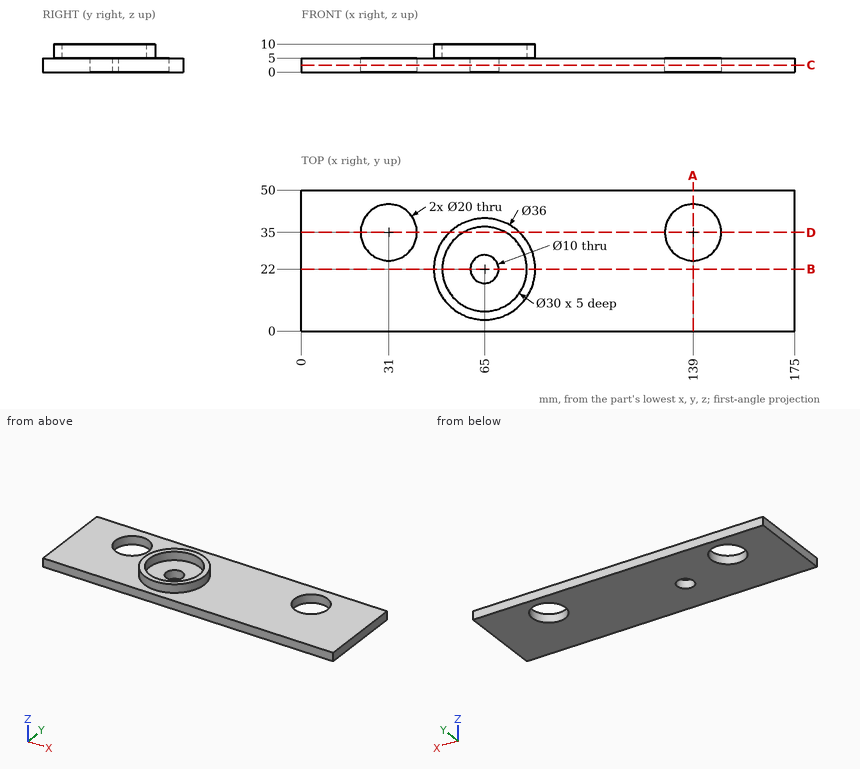
Check sheet for the drawn part. Datum: minimum x, y, z corner. Units: mm. Coordinates: 2 decimals unless noted, no trailing zeros. Write each loop counter-clockwise with the first axis right and the second up, starting at its lowest first coordinate (ties: lowest second). Pieces come first, ordered by that corner, then holes. Notation, with made-up numbers: M 49,-13.75 L 93,-13.75 A12 cw 93,4.25 Z; hole C 40.5,-6.5 d2. An arc over 180 degrees is marked long. One line per item, written item: value.
Item 1: Scan lines: line 1 along Y through (x, z) = (139, 3.75); line 2 along X through (y, z) = (21, 9.75); line 3 along Z through (x, y) = (72, 44.5). Record each from-to range of solid material in increasing order.
Check sheet entries:
line 1: y = 0 to 25, 45 to 50
line 2: x = 47.03 to 50.03, 79.97 to 82.97
line 3: z = 0 to 5
Item 2: Section check C-C, the plane z = 2.5. Record the boundary of the cut face in (x, y).
Check sheet entries:
outline: M 0,0 L 175,0 L 175,50 L 0,50 Z; hole C 31,35 d20; hole C 65,22 d10; hole C 139,35 d20
Item 3: Section check B-B, the plane y = 22. Record the boundary of the cut face in (x, z).
Check sheet entries:
outline: M 0,0 L 60,0 L 60,5 L 50,5 L 50,10 L 47,10 L 47,5 L 0,5 Z; M 70,0 L 175,0 L 175,5 L 83,5 L 83,10 L 80,10 L 80,5 L 70,5 Z
Item 4: Section check A-A, the plane x = 139. Record the boundary of the cut face in (y, z), plus the area to 3 significant figures.
Check sheet entries:
outline: M 0,0 L 25,0 L 25,5 L 0,5 Z; M 45,0 L 50,0 L 50,5 L 45,5 Z
area: 150 mm^2
Item 5: Section check D-D, the plane y = 35. Record the boundary of the cut face in (x, z), plus the area to 3 significant figures.
Check sheet entries:
outline: M 0,0 L 21,0 L 21,5 L 0,5 Z; M 41,0 L 129,0 L 129,5 L 77.45,5 L 77.45,10 L 72.48,10 L 72.48,5 L 57.52,5 L 57.52,10 L 52.55,10 L 52.55,5 L 41,5 Z; M 149,0 L 175,0 L 175,5 L 149,5 Z
area: 725 mm^2
Item 6: Gauge pin test, flat end, axial feed: pin 1 Ø23 at (x, y) = (31, 35) entering from +Z. Record the tip position at first contact, or that the pin passes through.
Check sheet entries:
pin 1: stops at z = 5
